The drawing under review shows one solid part. Ordinate dimensions are in mm from its lowest x, y, z. Give positions to 0.01 mm unless a question says otherwise; leave off trailing zeros. Write each loop counter-clockwise with the first axis right and the second up, starting at its lowest first coordinate (ties: lowest second). Pieces come first, ordered by that corner, then holes. Notation, with made-up numbers: (18, -32) -> (54, -32) arc R18 ccw to (54, -27) -> close; hole circle Ø5 at (69.25, 71.5). An arc over 180 degrees is marked (long way). Answer as a JSON object with one key per item and string values.
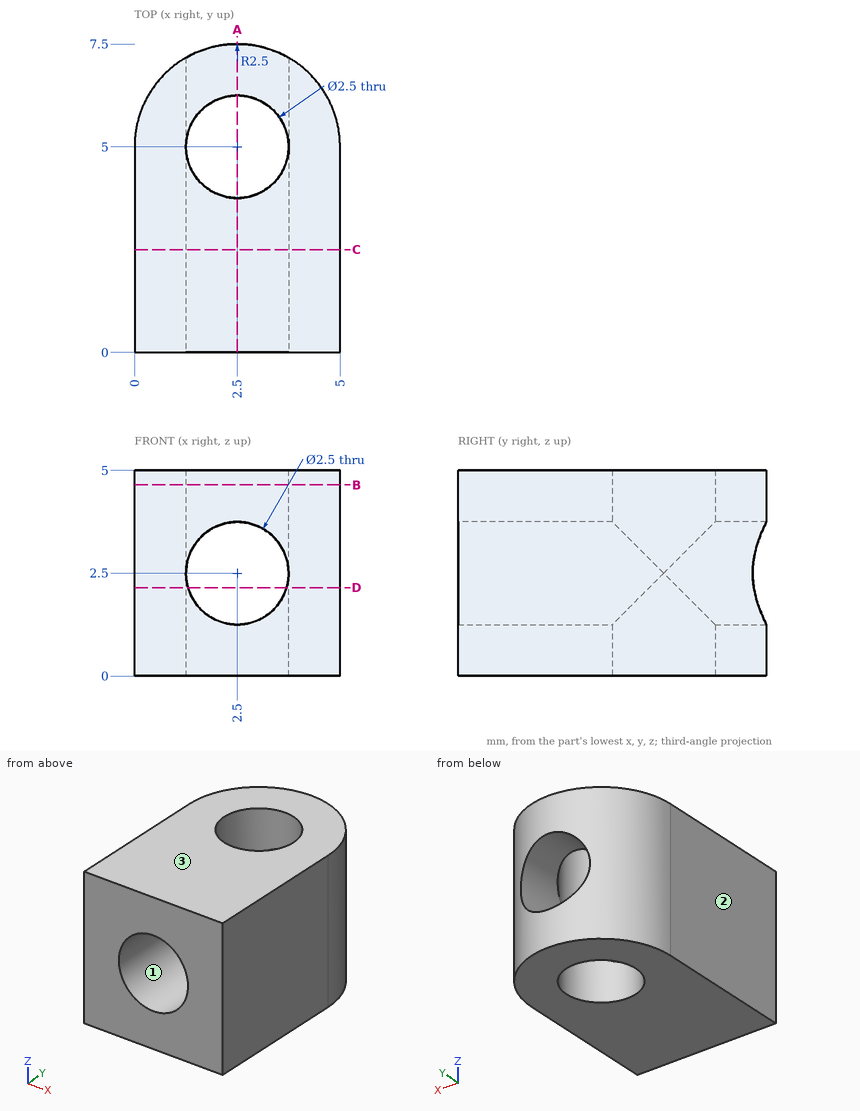
(1) Clearance check with flat-ended pins moving along their axes: pin 1 (3 mm diameter, centred on x = 2.5, y = 5, fed in from -Z); pin 2 (1.5 mm diameter, centred on x = 4, z = 1.5, fed in from +Y). State where each tip first meets the part, or that it passes through.
Here are the results:
{"pin 1": "stops at z = 0", "pin 2": "stops at y = 7.38"}
(2) The part is to be moulded in two halves that separate along Z. For the marked faces 1, 2 and 3, say which applies: +Z half, -Z half, draft (parallel to the pull), parting line (faces both ways), or undercut.
Here are the results:
{"face 1": "undercut", "face 2": "draft", "face 3": "+Z half"}
(3) We need section C-C, the plane y = 2.5. State the section outline as (x, z) points.
Here are the results:
{"outline": "(0, 0) -> (5, 0) -> (5, 5) -> (0, 5) -> close; hole circle Ø2.5 at (2.5, 2.5)"}
(4) We need section D-D, the plane z = 2.15. State the section outline as (x, y) points, then the cut area to 3 significant figures.
Here are the results:
{"outline": "(0, 0) -> (1.3, 0) -> (1.3, 4.65) arc R1.25 cw to (1.3, 5.35) -> (1.3, 7.19) arc R2.5 ccw to (0, 5) -> close; (3.7, 0) -> (5, 0) -> (5, 5) arc R2.5 ccw to (3.7, 7.19) -> (3.7, 5.35) arc R1.25 cw to (3.7, 4.65) -> close", "area": "17.0 mm²"}
(5) We need section A-A, the plane x = 2.5. State the section outline as (y, z) points.
Here are the results:
{"outline": "(0, 0) -> (3.75, 0) -> (3.75, 1.25) -> (0, 1.25) -> close; (0, 3.75) -> (3.75, 3.75) -> (3.75, 5) -> (0, 5) -> close; (6.25, 0) -> (7.5, 0) -> (7.5, 1.25) -> (6.25, 1.25) -> close; (6.25, 3.75) -> (7.5, 3.75) -> (7.5, 5) -> (6.25, 5) -> close"}
(6) We need section B-B, the plane z = 4.65. State the section outline as (x, y) points, then the cut area to 3 significant figures.
Here are the results:
{"outline": "(0, 0) -> (5, 0) -> (5, 5) arc R2.5 ccw to (0, 5) -> close; hole circle Ø2.5 at (2.5, 5)", "area": "29.9 mm²"}
(7) For line 1 along Y through (x, z) = (2.5, 4); line 2 along X through (y, z) = (5, 2.9), list the stretches that pass through material, from the lowest coordinate up.
Here are the results:
{"line 1": "y = 0 to 3.75, 6.25 to 7.5", "line 2": "x = 0 to 1.25, 3.75 to 5"}
